Job drawing, mm, ordinate dimensions from the low corner. One solid piece. A direction names the side the tool comes from. Coordinates: 2 decimals unless noted, no trailing zeros. Loops run counter-clockwise (first coordinate to the right, second up) from the corner with the lowest first, then second, coordinate; pieces in that order, holes last. Notation, with made-up numbers: (-5.75, -34) - (25.25, -34) arc R21 ccw to (25.25, -4) - close; hole circle Ø1 at (-29, 16.5). An arc over 180 degrees is marked (long way). Use a Markdown table: item, result. Add a question column.
1) Drop flat-ended pins along their axis: P1, Ø2, axis at x = 2.5, z = 12.5, coming from the -Y side; P2, Ø2, axis at x = 2, y = 2.5, coming from the +Z side. Give the stop position or say it passes through.
2) Tool access for the marked faces 1 and 2: list every direction of +Z, -Z, +X, -X, +Y, -Y with a clear straight run to the whole face (end or side of a thin tool).
3) Band-saw the part on D-D (z = 11.5). Give the cut face in (x, y).
4) Probe probe 1 along Z at (x, y) = (2.55, 2.7); probe 2 along Z at (x, y) = (2, 0.25); probe 3 along X at (y, z) = (2.2, 3.75). List the from-to ranges inside material, lowest first. Write a range as [from, to].
5) Band-saw the part on A-A (x = 1.9). Give the cut face in (y, z).
6) Band-saw the part on C-C (z = 4). Give the cut face in (x, y), plus the area to 3 significant figures.
7) Band-saw the part on B-B (y = 1.9). Give the cut face in (x, z).
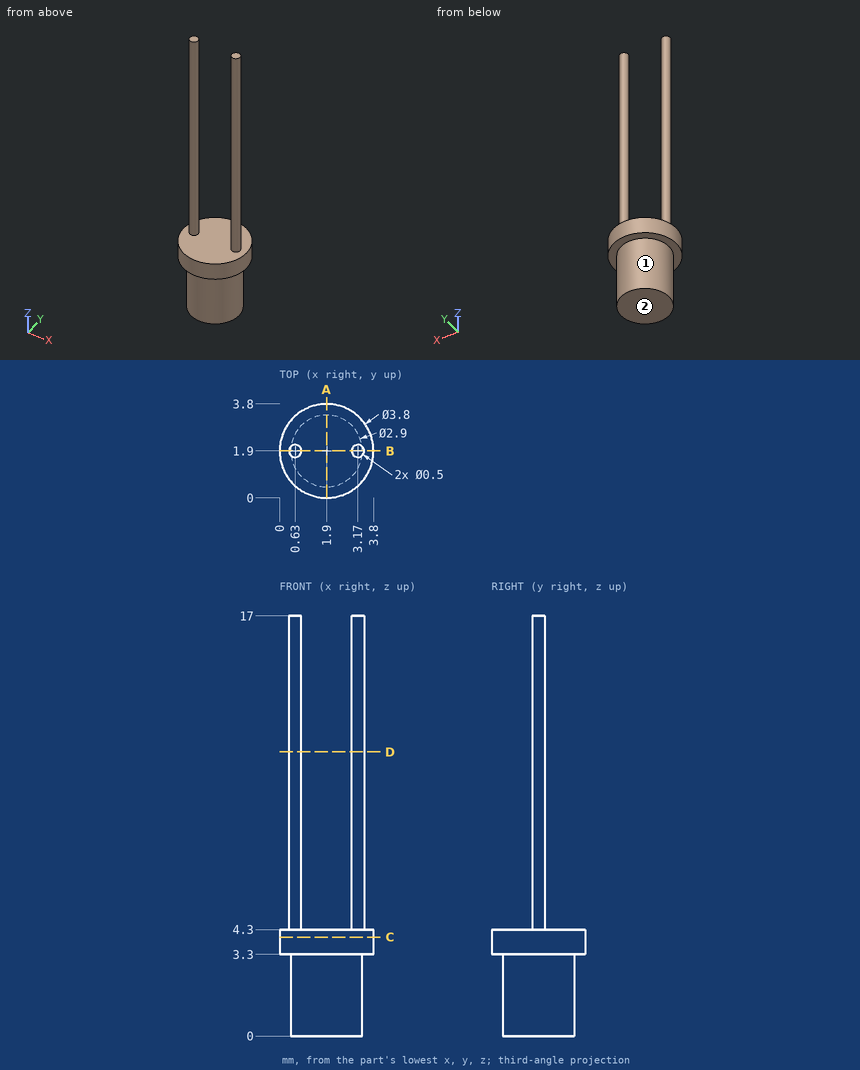
Answer block:
| question | item | result |
|---|---|---|
| 1 | P1 | y = 1.65 |
| 1 | P2 | z = 4.3 |
| 2 | face 1 | -Z |
| 2 | face 2 | -Z, +X, -X, +Y, -Y |
| 3 | outline | circle Ø0.5 at (0.63, 1.9); circle Ø0.5 at (3.17, 1.9) |
| 4 | probe 1 | [0, 4.3] |
| 4 | probe 2 | [3.3, 4.3] |
| 4 | probe 3 | [0.02, 3.78] |
| 5 | outline | (0, 3.3) - (0.45, 3.3) - (0.45, 0) - (3.35, 0) - (3.35, 3.3) - (3.8, 3.3) - (3.8, 4.3) - (0, 4.3) - close |
| 6 | outline | circle Ø3.8 at (1.9, 1.9) |
| 6 | area | 11.3 mm2 |
| 7 | outline | (0, 3.3) - (0.45, 3.3) - (0.45, 0) - (3.35, 0) - (3.35, 3.3) - (3.8, 3.3) - (3.8, 4.3) - (3.42, 4.3) - (3.42, 17) - (2.92, 17) - (2.92, 4.3) - (0.88, 4.3) - (0.88, 17) - (0.38, 17) - (0.38, 4.3) - (0, 4.3) - close |
